Geometry: final body of the model. Coordinates: model frame, mm. A direction names the side the tool comes from. Give positions to 0.01 mm unless a question says otherwise; leave off trailing zeros. Write each loop counter-clockwise with the first axis right and the second up, starting at its lowest first coordinate (ties: lowest second). Pieces come first, ordered by that corner, then holes. Notation, with made-up numbers: (79.5, -34) - (136.5, -34) arc R22 cw to (136.5, -11) - close; hole circle Ø6 at (55.25, -34). An arc over 180 degrees is marked (long way). Use CSV: the item, a comma, the result in double quotes. Start each with the question number.
(1) Section A-A on x = 0. Output: boundary loops of the cut face in (y, z).
(2) Section D-D on z = 2.5. Count the separate pieces of the cut face and the enclosed holes in it, and give its area (3 significant figures).
(3) Section C-C on y = -7. Output: boundary loops of the cut face in (x, z).
(4) Line query: probe 1 along Y at (x, z) = (0, 1.6); probe 2 along Y at (x, z) = (-4.25, 1.1); probe 3 along Y at (x, z) = (-7, 1.45). Output: solid intervals per line, ascending. Write a range as [from, to].
(5) Reachability of faces 1 (the cylindrical face through (-4.035, 6.167, 2.285)), 2 (the flat face through (5.2, 0.2, 3)), 3 (the cylindrical face through (-0.07, -10.05, 0.3)) from +Z, -Z, +X, -X, +Y, -Y: full face, straight path, thin tool, end or side. Return the list, or none.
(6) Section B-B on x = -5.75. Output: boundary loops of the cut face in (y, z), and give its area (3 significant figures).
(7) First-contact query: pin 1 Ø8 at (x, y) = (5.66, -5.66) entering from -Z; pin 2 Ø4.5 at (x, y) = (5.66, 5.66) entering from +Z; pin 3 Ø1.9 at (x, y) = (4.5, 4.5) entering from -Z; pin 4 Ø10 at (x, y) = (-3, -4) entering from -Z. Flat tips, straight axial feed; report the tip coordinate or a pass-through.
from build123d import *

# Parameters (mm, degrees)
D24_D6_5_R                      = 12
D24_D6_5_R_2                    = 3.25
D24_3_D6_5_DEPTH                = 3
EXTRUDE_START                   = 3
SKETCH_D9_8_1_5_R               = 4.9
SKETCH_D9_8_1_5_R_2             = 3.25
EXTRUDE_D9_8_1_5_DEPTH          = 1.5
F_4XD3_4_D6_3_PCD16_D           = 3.4
F_4XD3_4_D6_3_PCD16_CBORE_D     = 6.3
F_4XD3_4_D6_3_PCD16_CBORE_DEPTH = 1.55
SKETCH_1093_R                   = 10.05
CUT_EXTRUDE_D20_1_0_6_DEPTH     = 0.6
F_4XM2X0_4_PCD14_D              = 1.6


with BuildPart() as part:
    # 转接板_D24_工具通孔D6.5_截面 → 转接板_D24_厚3_工具通孔D6.5 (new body)
    with BuildSketch(Plane.XY):
        Circle(D24_D6_5_R)
        Circle(D24_D6_5_R_2, mode=Mode.SUBTRACT)
    extrude(amount=D24_3_D6_5_DEPTH)

    # 轴承内孔定位台_D9.8_高1.5_截面 → 轴承内孔定位台_D9.8_高1.5 (add)
    with BuildSketch(Plane.XY.offset(EXTRUDE_START)):
        Circle(SKETCH_D9_8_1_5_R)
        Circle(SKETCH_D9_8_1_5_R_2, mode=Mode.SUBTRACT)
    extrude(amount=EXTRUDE_D9_8_1_5_DEPTH)

    # 轴承内圈_4xD3.4通孔_D6.3平底沉孔_PCD16 (through all)
    with Locations(Plane(origin=(5.656854249, -5.656854249, 0), x_dir=(-1, 0, 0), z_dir=(0, 0, -1))):
        with Locations((0, 0), (11.313708498, 0), (11.313708498, 11.313708498), (0, 11.313708498)):
            CounterBoreHole(F_4XD3_4_D6_3_PCD16_D / 2, F_4XD3_4_D6_3_PCD16_CBORE_D / 2, F_4XD3_4_D6_3_PCD16_CBORE_DEPTH)

    # Sketch 1093 → 原舵盘定位槽_D20.1_深0.6 (cut)
    with BuildSketch(Plane.XY):
        Circle(SKETCH_1093_R)
    extrude(amount=CUT_EXTRUDE_D20_1_0_6_DEPTH, mode=Mode.SUBTRACT)

    # 原舵盘_4xM2x0.4通螺纹_PCD14 (through all)
    with Locations(Plane(origin=(0, -7, 0.6), x_dir=(-1, 0, 0), z_dir=(0, 0, -1))):
        with Locations((0, 0), (7, 7), (0, 14), (-7, 7)):
            Hole(F_4XM2X0_4_PCD14_D / 2)


solid = part.part
Check values:
1,outline,"(-12, 0) - (-10.05, 0) - (-10.05, 0.6) - (-7.8, 0.6) - (-7.8, 3) - (-12, 3) - close; (-6.2, 0.6) - (-3.25, 0.6) - (-3.25, 4.5) - (-4.9, 4.5) - (-4.9, 3) - (-6.2, 3) - close; (3.25, 0.6) - (6.2, 0.6) - (6.2, 3) - (4.9, 3) - (4.9, 4.5) - (3.25, 4.5) - close; (7.8, 0.6) - (10.05, 0.6) - (10.05, 0) - (12, 0) - (12, 3) - (7.8, 3) - close"
2,separate pieces,"1"
2,enclosed holes,"9"
2,area,"375 mm²"
3,outline,"(-9.75, 0) - (-8.51, 0) - (-8.51, 1.55) - (-6.7, 1.55) - (-6.7, 3) - (-9.75, 3) - close; (-4.61, 1.55) - (-2.81, 1.55) - (-2.81, 0.6) - (-0.8, 0.6) - (-0.8, 3) - (-4.61, 3) - close; (0.8, 0.6) - (2.81, 0.6) - (2.81, 1.55) - (4.61, 1.55) - (4.61, 3) - (0.8, 3) - close; (6.7, 1.55) - (8.51, 1.55) - (8.51, 0) - (9.75, 0) - (9.75, 3) - (6.7, 3) - close"
4,probe 1,"y = [-12, -7.8], [-6.2, -3.25], [3.25, 6.2], [7.8, 12]"
4,probe 2,"y = [-11.22, -8.48], [-2.84, 2.84], [8.48, 11.22]"
4,probe 3,"y = [-9.75, -8.51], [-2.81, -0.8], [0.8, 2.81], [8.51, 9.75]"
5,face 1,"+Z, -Z"
5,face 2,"+Z"
5,face 3,"-Z"
6,outline,"(-10.53, 0) - (-8.81, 0) - (-8.81, 1.55) - (-7.35, 1.55) - (-7.35, 3) - (-10.53, 3) - close; (-3.96, 1.55) - (-2.51, 1.55) - (-2.51, 0.6) - (2.51, 0.6) - (2.51, 1.55) - (3.96, 1.55) - (3.96, 3) - (-3.96, 3) - close; (7.35, 1.55) - (8.81, 1.55) - (8.81, 0) - (10.53, 0) - (10.53, 3) - (7.35, 3) - close"
6,area,"30.8 mm²"
7,pin 1,"stops at z = 0"
7,pin 2,"stops at z = 3"
7,pin 3,"stops at z = 1.55"
7,pin 4,"stops at z = 0.6"
